Geometry check sheet. Reference: the model listing, model coordinates, mm. A direction names the side the tool comes from. Round coordinates to 2 decimals unless told otherwise and drop trailing zeros. Order: outer loops, then holes, each group sorted by start corner. A loop starts at its lowest first (then second) coordinate and runs counter-clockwise, first axis right, second up.
(1) Cross-section at C-C on x = -35. Enter the section's corners in (y, z), and give its area (3 significant figures).
(2) Set-up check for faces 1 (the face through (10.35, -45.12, 3.13)), 2 (the face through (132, 60, 0)): record each of +Z, -Z, +X, -X, +Y, -Y from which the full face is reachable in a straight line by a thin tool's end or side.
(3) Draft check along Y on faces 3 (the face through (49.06, -128.344, 3.131)), 4 (the face through (43.5, 124.8, 3.1)), 5 (the face through (-53.234, -0.663, 3.131)), 6 (the face through (152.16, 45.12, 3.13)). Enter one of: pulls with the +Y half, pulls with the -Y half, needs draft (parallel to the pull), parting line crosses it, or undercut.
(4) Gauge pin test, flat ends, axial feed: P1, Ø2, axis at x = 47.5, z = 2.5, coming from the -Y side; P2, Ø1.9, axis at x = 72.5, z = 4, coming from the +Y side; P3, Ø1.9, axis at x = 77, z = 4.5, coming from the -Y side. Record the tip position at first contact, or that the pin passes through.
(5) Thickness scan on L1, parallel to Y at x = 194.5, z = 4.5; L2, parallel to Y at x = 114, z = 5; L3, parallel to X at y = -74.5, z = 4.5. Record the ranges inside material, lowest first.
(6) Cross-section at D-D on y = -93. Enter the section's corners in (x, z), and give its area (3 significant figures).
(7) Cross-section at A-A on z = 4.5. Enter the section's corners in (x, y), and give its area (3 significant figures).
(8) Cross-section at B-B on x = 90.5. Enter the section's corners in (y, z), and give its area (3 significant figures).
from build123d import *

# Parameters (mm, degrees)
BOSS_EXTRUDE1_DEPTH = 6.35
CUT_EXTRUDE1_DEPTH  = 7.35
SKETCH3_OUTSIDE_W   = 609.496
SKETCH3_OUTSIDE_H   = 769.968
CUT_EXTRUDE6_DEPTH  = 7.35


with BuildPart() as part:
    # Sketch1 → Boss-Extrude1 (new body)
    with BuildSketch(Plane.XY):
        Polygon((228.232926514, 307.505861177), (-209.583790114, 0.94329584), (-209.583790114, -0.94329584), (228.232926514, -307.505861177), (244.956408235, -271.642238892), (244.956408235, 271.642238892), align=None)
    extrude(amount=BOSS_EXTRUDE1_DEPTH)

    # Sketch2 → Cut-Extrude1 (cut, through all)
    with BuildSketch(Plane(origin=(0, 0, 0), x_dir=(-1, 0, 0), z_dir=(0, 0, -1))):
        with BuildLine():
            Line((-46.185656441, -54.927437645), (26.505438481, -35.03371061))
            ThreePointArc((26.505438481, -35.03371061), (53.239591757, 0), (26.505438481, 35.03371061))
            Line((26.505438481, 35.03371061), (-46.185656445, 54.927437638))
            Line((-46.185656445, 54.927437638), (-116.321160011, 54.927437643))
            Line((-116.321160011, 54.927437643), (-189.012254957, 35.03371061))
            ThreePointArc((-189.012254957, 35.03371061), (-215.746408235, 1e-09), (-189.012254959, -35.033710609))
            Line((-189.012254959, -35.033710609), (-116.32116001, -54.927437641))
            Line((-116.32116001, -54.927437641), (-46.185656441, -54.927437645))
        make_face()
    extrude(amount=-CUT_EXTRUDE1_DEPTH, mode=Mode.SUBTRACT)

    # Sketch3 outside → Cut-Extrude6 (cut, through all)
    with BuildSketch(Plane.XY):
        with Locations((17.686, 0)):
            Rectangle(SKETCH3_OUTSIDE_W, SKETCH3_OUTSIDE_H)
        Polygon((244.956408235, -253.143950628), (-152.4, 0), (244.956408235, 253.143950628), align=None, mode=Mode.SUBTRACT)
    extrude(amount=CUT_EXTRUDE6_DEPTH, mode=Mode.SUBTRACT)


solid = part.part
Found:
1. outline: (-74.79, 0) - (-31.5, 0) - (-31.5, 6.35) - (-74.79, 6.35) - close; (31.5, 0) - (74.79, 0) - (74.79, 6.35) - (31.5, 6.35) - close
1. area: 550 mm2
2. face 1: +Z, -Z
2. face 2: -Z, +X, -X, +Y, -Y
3. face 3: pulls with the -Y half
3. face 4: pulls with the +Y half
3. face 5: undercut
3. face 6: undercut
4. P1: stops at y = -127.99
4. P2: stops at y = 143.88
4. P3: stops at y = -146.75
5. L1: y = -221 to -33.05, 33.05 to 221
5. L2: y = -169.72 to -54.93, 54.93 to 169.72
5. L3: x = -35.46 to 244.96
6. outline: (-6.42, 0) - (244.96, 0) - (244.96, 6.35) - (-6.42, 6.35) - close
6. area: 1,600 mm2
7. outline: (-152.4, 0) - (244.96, -253.14) - (244.96, 253.14) - close; hole (-26.51, -35.03) - (46.19, -54.93) - (116.32, -54.93) - (189.01, -35.03) arc R36.32 ccw to (189.01, 35.03) - (116.32, 54.93) - (46.19, 54.93) - (-26.51, 35.03) arc R36.32 ccw to start
7. area: 77,000 mm2
8. outline: (-154.74, 0) - (-54.93, 0) - (-54.93, 6.35) - (-154.74, 6.35) - close; (54.93, 0) - (154.74, 0) - (154.74, 6.35) - (54.93, 6.35) - close
8. area: 1,270 mm2
